Read the model definition and answer for the solid it produces. Units are mm, in the model's axes. A direction names the side the tool comes from. Give positions to 0.01 mm unless a question says otherwise; leave off trailing zeros. Order: outer loops, then holes, each group sorted by start corner. A loop starts at its lowest first (then second) coordinate and runs counter-clockwise, first axis right, second up. Notation, with made-up numbers: M 44,85.25 L 50,85.25 A22 cw 50,113.25 Z; hole C -28.75,28.25 d3. An arc over 180 degrees is marked long. One line per item, written item: value.
from build123d import *

# Parameters (mm, degrees)
F1_DEPTH = 30
F2_R     = 4.4
F3_R     = 4.4
F4_DEPTH = 25
F5_R     = 2
F6_R     = 2


# Not quite as in the source:
# - a feature names something its author has since deleted; it is built from what else it names


with BuildPart() as f1:
    # F0 (on Front) → F1 (new body)
    with BuildSketch(Plane.XZ):
        Polygon((90, -1), (90, 1), (70, 1), (70, 44), (-70, 44), (-70, 1), (-90, 1), (-90, -1), (-68, -1), (-68, 42), (68, 42), (68, -1), align=None)
    extrude(amount=F1_DEPTH)

    # F2 (on face) + F3 (on face) → F4 (cut)
    with BuildSketch(Plane.XY.offset(1)):
        with Locations((-80, -15)):
            Circle(F2_R)
        with Locations((80, -15)):
            Circle(F2_R)
    with BuildSketch(Plane.XY.offset(44)):
        with Locations((-25, -15)):
            Circle(F3_R)
        with Locations((25, -15)):
            Circle(F3_R)
    extrude(amount=-F4_DEPTH, mode=Mode.SUBTRACT)

    # F5
    f5_edges = [f1.edges().sort_by_distance(p)[0] for p in [
        (-70, -15, 44),
        (70, -15, 44),
    ]]
    fillet(f5_edges, radius=F5_R)

    # F6
    f6_edges = [f1.edges().sort_by_distance(p)[0] for p in [
        (68, -15, -1),
        (-68, -15, -1),
    ]]
    fillet(f6_edges, radius=F6_R)


solid = f1.part
1) Determine the mould class of faces 6 (the face through (75, -15, -1)), 7 (the face through (27.365, -11.29, 43.014)), 8 (the face through (0, 0, 43)) for opening direction Y: +Y half, -Y half, draft (parallel to the pull), parting line (faces both ways), or undercut.
Reported:
face 6: draft
face 7: undercut
face 8: +Y half
2) Each of these flat-tipped pins is pushed along its axis until it touches: pin 1 Ø10 at (x, y) = (83, -22.5) entering from +Z; pin 2 Ø5 at (x, y) = (-32.5, -26) entering from -Z; pin 3 Ø15 at (y, z) = (-10.5, 28.5) entering from -X; pin 4 Ø5.5 at (x, y) = (25, -15) entering from +Z. Where does it stop, or does it pass through?
Reported:
pin 1: stops at z = 1
pin 2: stops at z = 42
pin 3: stops at x = -70
pin 4: passes through
3) Consider probe 1 along X at (y, z) = (-27.75, 24); probe 2 along Y at (x, z) = (-25, 43); probe 3 along Z at (x, y) = (12, -9). Determine where each line is inside the solid, lowest interval first.
Reported:
probe 1: x = -70 to -68, 68 to 70
probe 2: y = -30 to -19.4, -10.6 to 0
probe 3: z = 42 to 44
4) Find section D-D, the plane x = -56. Write down the section's boundary in (y, z).
Reported:
outline: M -30,42 L 0,42 L 0,44 L -30,44 Z
5) Which of the six approach directions +Z, -Z, +X, -X, +Y, -Y give full straight-line access (tool end or side, diameter ignored) to faces 1 (the face through (85, -15, 1)), 2 (the face through (-70, -15, 22)), 3 (the face through (75.604, -14.807, 0.014)), 4 (the face through (-85, -15, -1)), 5 (the face through (-1, -15, 42))?
Reported:
face 1: +Z, +X, +Y, -Y
face 2: +Z, -X, +Y, -Y
face 3: +Z, -Z
face 4: -Z, +X, -X, +Y, -Y
face 5: -Z, +Y, -Y
6) Find section C-C, the plane z = 34. Write down the section's boundary in (x, y).
Reported:
outline: M -70,-30 L -68,-30 L -68,0 L -70,0 Z; M 68,-30 L 70,-30 L 70,0 L 68,0 Z
7) Find section A-A, the plane y = -15. Count the separate pieces of the cut face and the enclosed holes in it, plus the area to 3 significant figures.
Reported:
separate pieces: 5
enclosed holes: 0
area: 458 mm^2
8) Find section B-B, the plane x = 80. Write down the section's boundary in (y, z).
Reported:
outline: M -30,-1 L -19.4,-1 L -19.4,1 L -30,1 Z; M -10.6,-1 L 0,-1 L 0,1 L -10.6,1 Z
